For this review, take the finished solid that the model builds, in its own axes (mm). Face numbers are marked on the shaded views. A direction names the side the tool comes from. Round coordinates to 2 decimals unless told otherwise and drop trailing zeros. Write each loop counter-clockwise with the first axis right and the second up, starting at its lowest first coordinate (ties: lowest second). Pieces come first, ordered by that corner, then holes. Notation, with made-up numbers: (-27, 68.5) -> (26, 68.5) arc R13 ccw to (26, 86.5) -> close; hole circle Ø11 at (-25, 15.25). An arc over 180 degrees is marked (long way). Answer as CSV lines item,"result". Start each with the question number.
Item 1: For pin 1 Ø1 at (x, y) = (5, -11.5) entering from +Z; pin 2 Ø2 at (x, y) = (0.5, -6.5) entering from -Z, all flat-tipped, find the tip position at first contact; note any pin that passes through.
Item 2: Take a section at A-A on x = 0. Give the boundary of the cut face in (y, z), then the cut area to 3 significant figures.
Item 3: Machinability: for the marked faces 1 and 2, which of the approach directions +Z, -Z, +X, -X, +Y, -Y give a long, thin tool a straight path to every point of the face, cutting with its end or side? Answer none if there is none.
Item 4: Mouldability with a two-part tool opening along Z and no side actions: class the marked faces 3, 4 and 5 as +Z half, -Z half, draft (parallel to the pull), parting line (faces both ways), or undercut.
Item 5: Wall thickness on probe 1 along Z at (x, y) = (0, -3); probe 2 along Y at (x, z) = (5, -0.5); probe 3 along Z at (x, y) = (0, -11): over which ranges is each line inside the solid? List them lowest first. Write a range as from..to.
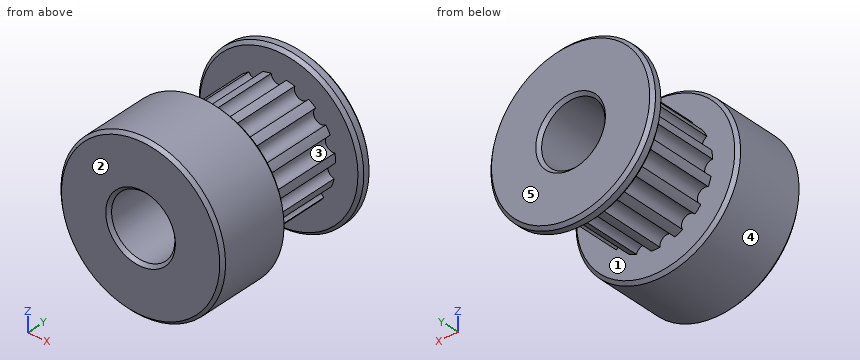
```python
from build123d import *

# Parameters (mm, degrees)
F0_R     = 6.5
F1_DEPTH = 1
F2_R     = 4.5
F3_DEPTH = 7
F4_R     = 6.5
F5_DEPTH = 6
F6_R     = 0.6
F7_DEPTH = 7
F8_R     = 2.5
F9_DEPTH = 14.001
F10_SIZE = 0.25


with BuildPart() as f1:
    # F0 (on Front) → F1 (new body)
    with BuildSketch(Plane.XZ):
        Circle(F0_R)
    extrude(amount=F1_DEPTH)

    # F2 (on face) → F3 (join)
    with BuildSketch(Plane.XZ.offset(1)):
        Circle(F2_R)
    extrude(amount=F3_DEPTH)

    # F4 (on face) → F5 (join)
    with BuildSketch(Plane.XZ.offset(8)):
        Circle(F4_R)
    extrude(amount=F5_DEPTH)

    # F6 (on face) → F7 (cut, through all)
    with BuildSketch(Plane.XZ.offset(1)):
        with Locations((0, 4.5)):
            Circle(F6_R)
        with Locations((-1.830315, 4.110955)):
            Circle(F6_R)
        with Locations((-3.344152, 3.011088)):
            Circle(F6_R)
        with Locations((-4.279754, 1.390576)):
            Circle(F6_R)
        with Locations((-4.475349, -0.470378)):
            Circle(F6_R)
        with Locations((-3.897114, -2.25)):
            Circle(F6_R)
        with Locations((-2.645034, -3.640576)):
            Circle(F6_R)
        with Locations((-0.935603, -4.401664)):
            Circle(F6_R)
        with Locations((0.935603, -4.401664)):
            Circle(F6_R)
        with Locations((2.645034, -3.640576)):
            Circle(F6_R)
        with Locations((3.897114, -2.25)):
            Circle(F6_R)
        with Locations((4.475349, -0.470378)):
            Circle(F6_R)
        with Locations((4.279754, 1.390576)):
            Circle(F6_R)
        with Locations((3.344152, 3.011088)):
            Circle(F6_R)
        with Locations((1.830315, 4.110955)):
            Circle(F6_R)
    extrude(amount=F7_DEPTH, mode=Mode.SUBTRACT)

    # F8 (on face) → F9 (cut, through all)
    with BuildSketch(Plane.XZ.offset(14)):
        Circle(F8_R)
    extrude(amount=-F9_DEPTH, mode=Mode.SUBTRACT)

    # F10
    f10_edges = [f1.edges().sort_by_distance(p)[0] for p in [
        (6.5, -11, 0),
        (-6.5, -8, 0),
        (-6.5, -14, 0),
        (6.5, -0.5, 0),
        (-6.5, 0, 0),
        (-6.5, -1, 0),
        (-2.5, -14, 0),
        (2.5, -7, 0),
        (-2.5, 0, 0),
    ]]
    chamfer(f10_edges, length=F10_SIZE)


solid = f1.part
```
Output values:
1,pin 1,"stops at z = 4.69"
1,pin 2,"stops at z = -4.5"
2,outline,"(-14, -6.25) -> (-13.75, -6.5) -> (-8.25, -6.5) -> (-8, -6.25) -> (-8, -4.5) -> (-1, -4.5) -> (-1, -6.25) -> (-0.75, -6.5) -> (-0.25, -6.5) -> (0, -6.25) -> (0, -2.75) -> (-0.25, -2.5) -> (-13.75, -2.5) -> (-14, -2.75) -> close; (-14, 2.75) -> (-13.75, 2.5) -> (-0.25, 2.5) -> (0, 2.75) -> (0, 6.25) -> (-0.25, 6.5) -> (-0.75, 6.5) -> (-1, 6.25) -> (-1, 3.9) -> (-8, 3.9) -> (-8, 6.25) -> (-8.25, 6.5) -> (-13.75, 6.5) -> (-14, 6.25) -> close"
2,area,"79.4 mm^2"
3,face 1,"none"
3,face 2,"+Z, -Z, +X, -X, -Y"
4,face 3,"undercut"
4,face 4,"parting line"
4,face 5,"draft"
5,probe 1,"z = -4.5..-2.5, 2.5..3.9"
5,probe 2,"y = -14..-8, -1..0"
5,probe 3,"z = -6.5..-2.5, 2.5..6.5"
